Print and shaded views of the part. All mm, measured from the part's lowest x, y and z. A direction names the side the tool comes from. Round coordinates to 2 decimals unless told otherwise and drop trailing zeros. Loops run counter-clockwise (first coordinate to the right, second up) from the corner with the lowest first, then second, coordinate; pieces in that order, holes last. Notation, with made-up numbers: (-38, 15) - (16, 15) arc R9 cw to (16, 28) - close; hole circle Ø8 at (65, 78.25). An arc over 180 degrees is marked (long way). Put each result on its own line as item: value. Start each with the question number.
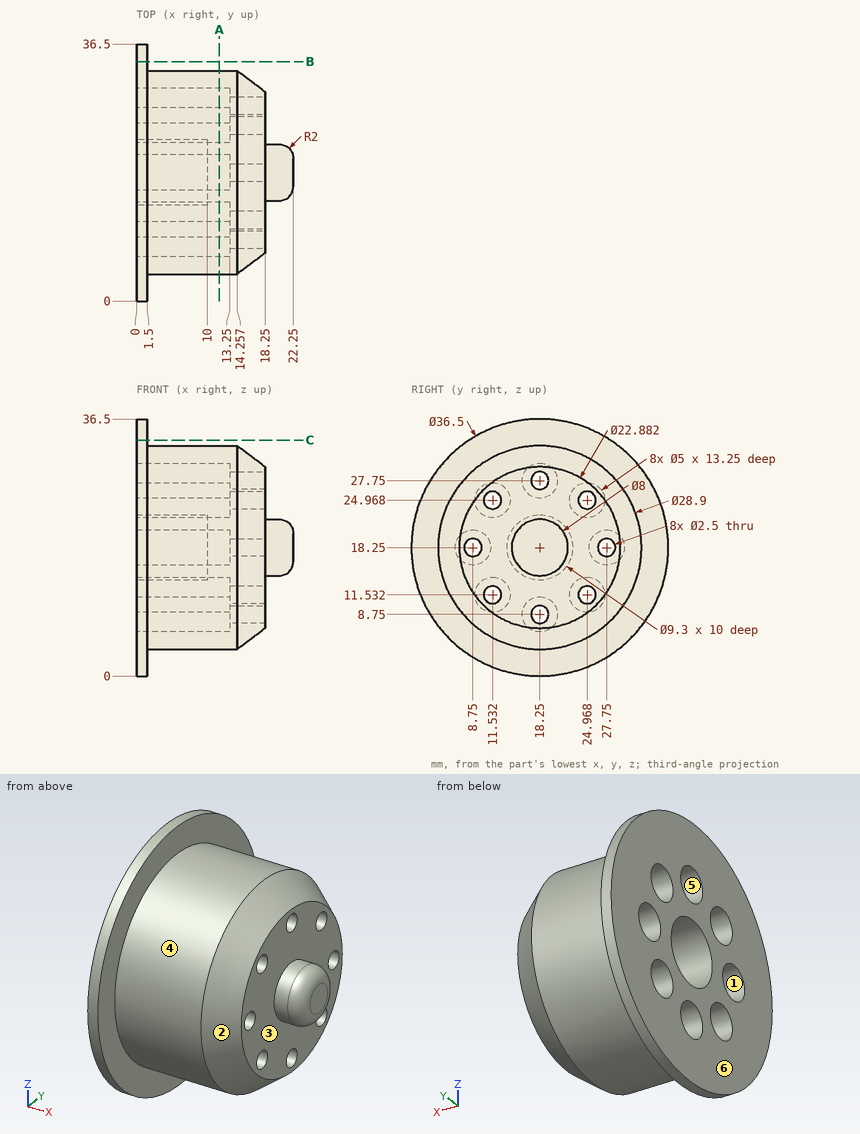
Item 1: Slice it at B-B (y = 34). Give the cut face in (x, z).
Item 2: Which spindle directions (+Z, -Z, +X, -X, +Y, -Y) get a long thin tool onto all of the face, cutting with end or side? Do the marked faces 4, 5 and 6. Say none if no direction does.
Item 3: Two-plate mould, pull along Y, no slides. Class the marked faces 1, 2 and 3: pulls with the +Y half, pulls with the -Y half, needs draft (parallel to the pull), parting line crosses it, or undercut.
Item 4: Drop flat-ended pins along their axis: pin 1 Ø8 at (x, y) = (8, 10) entering from -Z; pin 2 Ø4 at (y, z) = (11.53, 24.97) entering from +X; pin 3 Ø2.5 at (y, z) = (12, 24) entering from -X; pin 4 Ø2 at (y, z) = (18.25, 27.75) entering from -X (3 decimals). Give the stop position or say it passes through.
Item 5: Slice it at A-A (x = 11.75). Give the number of separate pieces and of enclosed holes in the cut face, plus the area to 3 significant figures.
Item 6: Slice it at C-C (z = 33.5). Give the cut face in (x, y) (1 decimal).
Item 7: Drill centre lines: probe 1 along Z at (x, y) = (9.75, 24) (1 decimal); probe 2 along Z at (x, y) = (4, 10.5) (1 decimal); probe 3 along X at (y, z) = (11, 4). Where is each one in solid material? Low to high. Write a range as [from, to].
Computed values:
1. outline: (0, 9.03) - (1.5, 9.03) - (1.5, 27.47) - (0, 27.47) - close
2. face 4: +X
2. face 5: -X
2. face 6: +Z, -Z, -X, +Y, -Y
3. face 1: undercut
3. face 2: parting line crosses it
3. face 3: needs draft
4. pin 1: stops at z = 4.44
4. pin 2: stops at x = 18.25
4. pin 3: stops at x = 13.25
4. pin 4: passes through
5. separate pieces: 1
5. enclosed holes: 8
5. area: 499 mm^2
6. outline: (0, 8.2) - (1.5, 8.2) - (1.5, 28.3) - (0, 28.3) - close
7. probe 1: z = [5, 9.2], [13.8, 22.7], [27.3, 31.5]
7. probe 2: z = [6.1, 9.3], [13.8, 16.5], [20, 22.7], [27.2, 30.4]
7. probe 3: x = [0, 1.5]
